```python
from build123d import *

# Parameters (mm, degrees)
BASPROSKE_W         = 15
BASPROSKE_H         = 13.2
TOOTHCUT_DEPTH      = 24.947442452
TEETHCUTS_COUNT     = 20
TEETHCUTS_ANGLE     = 342
BORSKE_R            = 4
BORE_DEPTH          = 50.0000508
BOSS_EXTRUDE1_START = -15
BOSS_EXTRUDE1_DEPTH = 15
SKETCH2_R           = 7.2
SKETCH2_R_2         = 6
CUT_EXTRUDE1_DEPTH  = 0.5
CUT_EXTRUDE2_DEPTH  = 2


with BuildPart() as part:
    # BasProSke → Base-Revolve (revolve)
    with BuildSketch(Plane(origin=(0, 0, 0), x_dir=(1, 0, 0), z_dir=(0, 1, 0)), mode=Mode.PRIVATE) as base_revolve_sk:
        with Locations((7.5, 6.6)):
            Rectangle(BASPROSKE_W, BASPROSKE_H)
    revolve(base_revolve_sk.sketch.rotate(Axis((-10, 0, 0), (1, 0, 0)), 180), axis=Axis((-10, 0, 0), (1, 0, 0)))

    # TooCutSke → ToothCut (cut, through all)
    with BuildSketch(Plane(origin=(0, 0, 0), x_dir=(0, 0, -1), z_dir=(1, 0, 0))):
        with BuildLine():
            ThreePointArc((0.599012827, 10.48189795), (0, 10.499), (-0.599012827, 10.48189795))
            ThreePointArc((-0.599012827, 10.48189795), (-0.986906343, 11.883983562), (-1.777012823, 13.105473306))
            ThreePointArc((-1.777012823, 13.105473306), (0, 13.2254), (1.777012823, 13.105473306))
            ThreePointArc((1.777012823, 13.105473306), (0.986906343, 11.883983562), (0.599012827, 10.48189795))
        make_face()
    toothcut = extrude(amount=TOOTHCUT_DEPTH, mode=Mode.SUBTRACT)

    # TeethCuts: ToothCut ×20 about axis
    teethcuts_axis = Axis((-10, 0, 0), (1, 0, 0))
    for i in range(1, TEETHCUTS_COUNT):
        add(toothcut.rotate(teethcuts_axis, i * TEETHCUTS_ANGLE / (TEETHCUTS_COUNT - 1)), mode=Mode.SUBTRACT)

    # BorSke → Bore (cut, symmetric)
    with BuildSketch(Plane(origin=(0, 0, 0), x_dir=(0, 0, -1), z_dir=(1, 0, 0))):
        with Locations(Location((0, 0, 0), (0, 0, 180))):
            Circle(BORSKE_R)
    extrude(amount=BORE_DEPTH, both=True, mode=Mode.SUBTRACT)

    # Sketch1 → Boss-Extrude1 (add)
    with BuildSketch(Plane.ZY.offset(BOSS_EXTRUDE1_START)):
        with BuildLine():
            Line((2.383385736, 3.212393568), (-3.25941874, 2.318661139))
            ThreePointArc((-3.25941874, 2.318661139), (-0.62573786, 3.950753362), (2.383385736, 3.212393568))
        make_face()
    extrude(amount=BOSS_EXTRUDE1_DEPTH)

    # Sketch2 → Cut-Extrude1 (cut)
    with BuildSketch(Plane.ZY):
        Circle(SKETCH2_R)
        Circle(SKETCH2_R_2, mode=Mode.SUBTRACT)
    extrude(amount=-CUT_EXTRUDE1_DEPTH, mode=Mode.SUBTRACT)

    # Sketch3 → Cut-Extrude2 (cut)
    with BuildSketch(Plane(origin=(15, 0, 0), x_dir=(0, 0, -1), z_dir=(1, 0, 0))):
        Polygon((-0.892330227, 7.685800395), (0.817285157, 7.685800395), (0.817285157, 7.1159286), (0.247413362, 7.1159286), (0.247413362, 4.510800395), (-0.322458432, 4.510800395), (-0.322458432, 7.1159286), (-0.892330227, 7.1159286), align=None)
    extrude(amount=-CUT_EXTRUDE2_DEPTH, mode=Mode.SUBTRACT)


solid = part.part
```
Read the model definition and answer for the solid it produces. Units are mm, in the model's axes. A direction names the side the tool comes from. Round coordinates to 2 decimals unless told otherwise and drop trailing zeros. Loops run counter-clockwise (first coordinate to the right, second up) from the corner with the lowest first, then second, coordinate; pieces in that order, holes last. Notation, with made-up numbers: (-15, 15) -> (43, 15) arc R14 cw to (43, 36) -> close; hole circle Ø8 at (-34, -25.5). An arc over 180 degrees is marked (long way). One line per item, written item: value.
1) Flat-ended cylindrical pins translate along their axes: P1, Ø2, axis at x = 6, z = 8.5, coming from the +Y side; P2, Ø0.6, axis at x = 14.5, y = 5.5, coming from the +Z side; P3, Ø8, axis at x = 12.5, z = 7, coming from the -Y side. Find the tip coordinate at first contact, or state that the pin passes through.
Answer list:
P1: stops at y = 9.55
P2: stops at z = 11.9
P3: stops at y = -11.9
2) A cutting plane is placed at C-C (z = 5). Determine the outline of the cut face in (x, y).
Answer list:
outline: (0, -11.38) -> (15, -11.38) -> (15, 11.38) -> (0, 11.38) -> (0, 5.18) -> (0.5, 5.18) -> (0.5, 3.32) -> (0, 3.32) -> (0, -3.32) -> (0.5, -3.32) -> (0.5, -5.18) -> (0, -5.18) -> close
3) A cutting plane is placed at B-B (y = -11). Determine the outline of the cut face in (x, z).
Answer list:
outline: (0, -6.29) -> (15, -6.29) -> (15, -4.61) -> (0, -4.61) -> close; (0, -2.76) -> (15, -2.76) -> (15, -0.69) -> (0, -0.69) -> close; (0, 0.69) -> (15, 0.69) -> (15, 2.76) -> (0, 2.76) -> close; (0, 4.61) -> (15, 4.61) -> (15, 6.29) -> (0, 6.29) -> close
4) Consider L1, parallel to Y at x = 2.25, z = 11; L2, parallel to X at y = 6.5, z = -0.5; L3, parallel to Z at x = 9.75, y = 4. Determine where each line is inside the solid, lowest interval first. Write a range as [from, to].
Answer list:
L1: y = [-6.29, -4.61], [-2.76, -0.69], [0.69, 2.76], [4.61, 6.29]
L2: x = [0.5, 15]
L3: z = [-10.16, 10.16]
5) The mould has two halves that part along Y. Classify faces 5 (the face through (7.395, 7.753, -9.016)), 6 (the face through (7.4, -10.5, 0)), 7 (the face through (7.395, 11.001, -4.614)): pulls with the +Y half, pulls with the -Y half, needs draft (parallel to the pull), parting line crosses it, or undercut.
Answer list:
face 5: undercut
face 6: pulls with the -Y half
face 7: pulls with the +Y half
6) For faces 1 (the face through (7.4, 9.04, -7.79)), 2 (the face through (7.4, -7.79, -9.04)), 3 (the face through (7.395, -8.489, 6.178)), 4 (the face through (7.395, -4.587, 10.971)), determine the directions among +Z, -Z, +X, -X, +Y, -Y from which every point of the face is accessible in a straight line to the end or side of a thin tool.
Answer list:
face 1: +X, -X, +Y
face 2: -Z, +X, -X
face 3: +X, -X
face 4: +Z, +X, -X
7) A cutting plane is placed at A-A (y = 0). Determine the outline of the cut face in (x, z), and give its area (3 significant figures).
Answer list:
outline: (0, -10.5) -> (15, -10.5) -> (15, -4) -> (0, -4) -> (0, -6) -> (0.5, -6) -> (0.5, -7.2) -> (0, -7.2) -> close; (0, 4) -> (15, 4) -> (15, 10.5) -> (0, 10.5) -> (0, 7.2) -> (0.5, 7.2) -> (0.5, 6) -> (0, 6) -> close
area: 194 mm²
